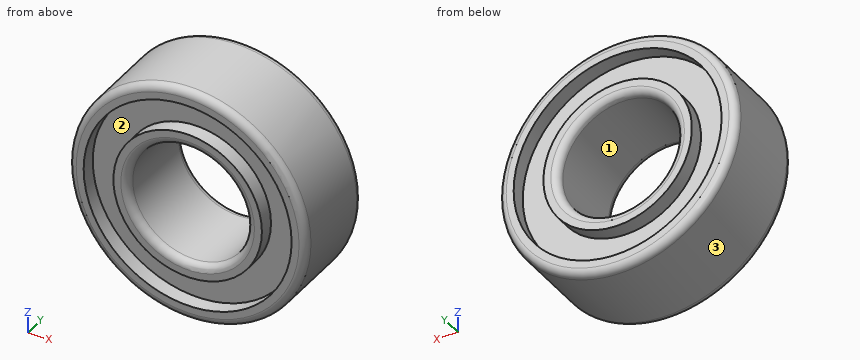
from build123d import *

# Parameters (mm, degrees)
F0_R     = 6.35
F0_R_2   = 3.175
F1_DEPTH = 2.3876
F2_R     = 5.55625
F2_R_2   = 3.96875
F3_DEPTH = 0.79375
F4_R     = 0.396875


# Not quite as in the source:
# - a pattern or mirror of a feature is missing from the dataset's text; its kind, count and spacing are read off the source's solid


with BuildPart() as f1:
    # F0 (on Front) → F1 (new body, symmetric)
    with BuildSketch(Plane.XZ):
        Circle(F0_R)
        Circle(F0_R_2, mode=Mode.SUBTRACT)
    extrude(amount=F1_DEPTH, both=True)

    # F2 (on face) → F3 (cut)
    with BuildSketch(Plane.XZ.offset(2.3876)):
        Circle(F2_R)
        Circle(F2_R_2, mode=Mode.SUBTRACT)
    f3 = extrude(amount=-F3_DEPTH, mode=Mode.SUBTRACT)

    # F3_copies: F3 across plane
    add(f3.mirror(Plane.ZX), mode=Mode.SUBTRACT)

    # F4
    f4_edges = [f1.edges().sort_by_distance(p)[0] for p in [
        (-3.175, -2.3876, 0),
        (3.175, 0, 0),
        (-3.175, 2.3876, 0),
        (-6.35, 2.3876, 0),
        (6.35, 0, 0),
        (-6.35, -2.3876, 0),
    ]]
    fillet(f4_edges, radius=F4_R)


solid = f1.part
Build history of the part. All positions in model axes, mm. Face numbers are marked on the shaded views. Coordinates: 2 decimals unless noted, no trailing zeros. Order: outer loops, then holes, each group sorted by start corner. A loop starts at its lowest first (then second) coordinate and runs counter-clockwise, first axis right, second up. Notation, with made-up numbers: (84.25, 53) - (105.25, 53) arc R9 ccw to (105.25, 67) - close; hole circle Ø4 at (46, 74.25). An arc over 180 degrees is marked (long way). Put each result on its own line as item: value.
1. Saw through at D-D (y = -0.8). Write the cut outline in (x, z) (3 decimals), and give its area (3 significant figures).
Answer sheet:
outline: circle Ø12.7 at (0, 0); hole circle Ø6.35 at (0, 0)
area: 95.0 mm^2
2. Probe line 1 along Z through (x, y) = (0, -1.75) (3 decimals); line 2 along Z through (x, y) = (-0.5, -1.9); line 3 along X through (y, z) = (1.85, -1.5). List the from-to ranges inside material, lowest first. Write a range as [from, to].
Answer sheet:
line 1: z = [-6.35, -5.556], [-3.969, -3.175], [3.175, 3.969], [5.556, 6.35]
line 2: z = [-6.33, -5.53], [-3.94, -3.14], [3.14, 3.94], [5.53, 6.33]
line 3: x = [-6.17, -5.35], [-3.67, -2.8], [2.8, 3.67], [5.35, 6.17]
3. Pull direction X, two halves, no side cores. Call the marked faces 1, 2 and 3: pulls with the +X half, pulls with the -X half, needs draft (parallel to the pull), parting line crosses it, or undercut.
Answer sheet:
face 1: undercut
face 2: undercut
face 3: parting line crosses it
4. Drop flat-ended pins along their axis: P1, Ø1, axis at y = 1.5, z = 3, coming from the -X side; P2, Ø1, axis at x = -2.5, y = -1, coming from the -Z side; P3, Ø2, axis at x = 1.5, y = 0.5, coming from the -Z side. Give the stop position or say it passes through.
Answer sheet:
P1: stops at x = -5.84
P2: stops at z = -6.03
P3: stops at z = -6.33
5. Saw through at C-C (y = 1.8). Give the number of separate pieces and of enclosed holes in the cut face, and give its area (3 significant figures).
Answer sheet:
separate pieces: 2
enclosed holes: 2
area: 47.5 mm^2
